Check sheet for the modelled part. Datum: model origin and axes. Units: mm. A direction names the side the tool comes from. Give positions to 0.01 mm unless a question says otherwise; leave off trailing zeros. Order: outer loops, then holes, each group sorted by start corner. A loop starts at its lowest first (then second) coordinate and runs counter-clockwise, first axis right, second up.
from build123d import *

# Parameters (mm, degrees)
IZIM1_R                     = 42
IZIM1_R_2                   = 40
Y_KSEKLIK_EKSTR_ZYON1_DEPTH = 15
IZIM2_R                     = 42
Y_KSEKLIK_EKSTR_ZYON2_DEPTH = 2
IZIM3_R                     = 1.75
KES_EKSTR_ZYON1_DEPTH       = 2
KES_EKSTR_ZYON2_DEPTH       = 2
Y_KSEKLIK_EKSTR_ZYON3_DEPTH = 7.5
Y_KSEKLIK_EKSTR_ZYON4_DEPTH = 35
Y_KSEKLIK_EKSTR_ZYON5_DEPTH = 4
Y_KSEKLIK_EKSTR_ZYON6_DEPTH = 4
IZIM9_W                     = 21
IZIM9_H                     = 3
Y_KSEKLIK_EKSTR_ZYON7_DEPTH = 45
IZIM10_R                    = 2.5
Y_KSEKLIK_EKSTR_ZYON8_DEPTH = 10
RADYUS1_R                   = 5


with BuildPart() as part:
    # Çizim1 → Yükseklik-Ekstrüzyon1 (new body)
    with BuildSketch(Plane(origin=(0, 0, 0), x_dir=(1, 0, 0), z_dir=(0, 1, 0))):
        with Locations(Location((0, 0, 0), (0, 0, 270))):
            Circle(IZIM1_R)
        with Locations(Location((0, 0, 0), (0, 0, 270))):
            Circle(IZIM1_R_2, mode=Mode.SUBTRACT)
    extrude(amount=Y_KSEKLIK_EKSTR_ZYON1_DEPTH)

    # Çizim2 → Yükseklik-Ekstrüzyon2 (add)
    with BuildSketch(Plane(origin=(0, 15, 0), x_dir=(1, 0, 0), z_dir=(0, 1, 0))):
        with Locations(Location((0, 0, 0), (0, 0, 270))):
            Circle(IZIM2_R)
    extrude(amount=Y_KSEKLIK_EKSTR_ZYON2_DEPTH)

    # Çizim3 → Kes-Ekstrüzyon1 (cut)
    with BuildSketch(Plane(origin=(0, 17, 0), x_dir=(1, 0, 0), z_dir=(0, 1, 0))):
        with Locations(Location((-13.5, 0, 0), (0, 0, 270))):
            Circle(IZIM3_R)
        with Locations(Location((13.5, 0, 0), (0, 0, 270))):
            Circle(IZIM3_R)
    extrude(amount=-KES_EKSTR_ZYON1_DEPTH, mode=Mode.SUBTRACT)

    # Çizim4 → Kes-Ekstrüzyon2 (cut)
    with BuildSketch(Plane(origin=(0, 17, 0), x_dir=(1, 0, 0), z_dir=(0, 1, 0))):
        with BuildLine():
            ThreePointArc((19.121323176, 19.121323176), (23.11330853, 20.564910887), (26.776285642, 18.419569137))
            ThreePointArc((26.776285642, 18.419569137), (30.026084807, -12.437211552), (5.909090909, -31.958295396))
            ThreePointArc((5.909090909, -31.958295396), (1.801989255, -30.88516514), (0, -27.041634566))
            ThreePointArc((0, -27.041634566), (1.156469426, -23.843623821), (4.090909091, -22.124973736))
            ThreePointArc((4.090909091, -22.124973736), (20.787289482, -8.610377228), (18.537428522, 12.752009403))
            ThreePointArc((18.537428522, 12.752009403), (17.677735465, 16.042240718), (19.121323176, 19.121323176))
        make_face()
    extrude(amount=-KES_EKSTR_ZYON2_DEPTH, mode=Mode.SUBTRACT)

    # Çizim5 → Yükseklik-Ekstrüzyon3 (add)
    with BuildSketch(Plane(origin=(0, 17, 0), x_dir=(1, 0, 0), z_dir=(0, 1, 0))):
        with BuildLine():
            Line((-10.5, -10), (-10.5, -2.645751311))
            ThreePointArc((-10.5, -2.645751311), (-9.5, 0), (-10.5, 2.645751311))
            Line((-10.5, 2.645751311), (-10.5, 18))
            Line((-10.5, 18), (10.5, 18))
            Line((10.5, 18), (10.5, 2.645751311))
            ThreePointArc((10.5, 2.645751311), (9.5, 0), (10.5, -2.645751311))
            Line((10.5, -2.645751311), (10.5, -10))
            Line((10.5, -10), (-10.5, -10))
        make_face()
    extrude(amount=Y_KSEKLIK_EKSTR_ZYON3_DEPTH)

    # Çizim6 → Yükseklik-Ekstrüzyon4 (add)
    with BuildSketch(Plane(origin=(0, 17, 0), x_dir=(1, 0, 0), z_dir=(0, 1, 0))):
        Polygon((-10.5, 18), (-10.5, 13), (-14.5, 13), (-14.5, 20), (-10.5, 20), align=None)
        Polygon((10.5, 20), (10.5, 18), (10.5, 13), (14.5, 13), (14.5, 20), align=None)
    extrude(amount=Y_KSEKLIK_EKSTR_ZYON4_DEPTH)

    # Çizim7 → Yükseklik-Ekstrüzyon5 (add)
    with BuildSketch(Plane(origin=(10.5, 0, 0), x_dir=(0, 0, -1), z_dir=(1, 0, 0))):
        Polygon((13, 52), (7.822875656, 17), (13, 17), align=None)
    extrude(amount=Y_KSEKLIK_EKSTR_ZYON5_DEPTH)

    # Çizim8 → Yükseklik-Ekstrüzyon6 (add)
    with BuildSketch(Plane.ZY.offset(10.5)):
        Polygon((-13, 52), (-7.822875656, 17), (-13, 17), align=None)
    extrude(amount=Y_KSEKLIK_EKSTR_ZYON6_DEPTH)

    # Çizim9 → Yükseklik-Ekstrüzyon7 (add)
    with BuildSketch(Plane(origin=(0, 17, 0), x_dir=(1, 0, 0), z_dir=(0, 1, 0))):
        with Locations((0, -16.5)):
            Rectangle(IZIM9_W, IZIM9_H)
    extrude(amount=Y_KSEKLIK_EKSTR_ZYON7_DEPTH)

    # Çizim10 → Yükseklik-Ekstrüzyon8 (add)
    with BuildSketch(Plane.XY.offset(18)):
        with Locations(Location((0, 54, 0), (0, 0, 180))):
            Circle(IZIM10_R)
    extrude(amount=Y_KSEKLIK_EKSTR_ZYON8_DEPTH)

    # Radyus1
    radyus1_edges = [part.edges().sort_by_distance(p)[0] for p in [
        (-10.5, 62, 16.5),
        (10.5, 62, 16.5),
    ]]
    fillet(radyus1_edges, radius=RADYUS1_R)


solid = part.part
1) Material ranges on L1, parallel to X at y = 16.25, z = 0; L2, parallel to X at y = 11.5, z = 0; L3, parallel to Y at x = 4.5, z = -11, recorded low to high.
Recorded:
L1: x = -42 to -15.25, -11.75 to 11.75, 15.25 to 22.5, 32.5 to 42
L2: x = -42 to -40, 40 to 42
L3: y = 15 to 24.5
2) Section check D-D, the plane x = -33. Record the cut outline in (y, z), then the cut area to 3 significant figures.
Recorded:
outline: (0, -25.98) - (17, -25.98) - (17, 25.98) - (0, 25.98) - (0, 22.61) - (15, 22.61) - (15, -22.61) - (0, -22.61) - close
area: 205 mm2
3) Section check A-A, the plane z = 0. Record the cut outline in (x, y), then the cut area to 4 significant figures.
Recorded:
outline: (-42, 0) - (-40, 0) - (-40, 15) - (-15.25, 15) - (-15.25, 17) - (-42, 17) - close; (-11.75, 15) - (11.75, 15) - (11.75, 17) - (9.5, 17) - (9.5, 24.5) - (-9.5, 24.5) - (-9.5, 17) - (-11.75, 17) - close; (15.25, 15) - (22.5, 15) - (22.5, 17) - (15.25, 17) - close; (32.5, 15) - (40, 15) - (40, 0) - (42, 0) - (42, 17) - (32.5, 17) - close
area: 336.5 mm2
4) Depth check by flat-ended pin: pin 1 Ø8 at (x, y) = (-1.5, 31.5) entering from -Z; pin 2 Ø6 at (y, z) = (19.5, 7) entering from -X; pin 3 Ø10.5 at (x, y) = (-3, 46.5) entering from +Z. Enter the tip coordinate at first touch or a pass-through.
Recorded:
pin 1: stops at z = 15
pin 2: stops at x = -41.66
pin 3: stops at z = 18
5) Set-up check for faces 1 (the face through (-10.5, 35, -16)), 2 (the face through (-13, 34, -20)), 3 (the face through (-10.5, 21, -6)), 4 (the face through (0, 54, 28)): record each of +Z, -Z, +X, -X, +Y, -Y from which the full face is reachable in a straight line by a thin tool's end or side.
Recorded:
face 1: -Z, +Y
face 2: -Z, +X, -X, +Y
face 3: +Z, -X, +Y
face 4: +Z, +X, -X, +Y
6) Draft check along Z on faces 5 (the face through (-12, 52, -17)), 6 (the face through (30.196, 16.014, 12.018)), 7 (the face through (-9.5, 20.7, 0)), 8 (the face through (12.472, 34.745, -10.448)). Enter one of: +Z half, -Z half, draft (parallel to the pull), parting line (faces both ways), or undercut.
Recorded:
face 5: draft
face 6: undercut
face 7: undercut
face 8: +Z half
7) Section check C-C, the plane y = 33. Record the cut outline in (x, z), then the cut area to 3 significant figures.
Recorded:
outline: (-14.5, -20) - (-10.5, -20) - (-10.5, -10.19) - (-14.5, -10.19) - close; (-10.5, 15) - (10.5, 15) - (10.5, 18) - (-10.5, 18) - close; (10.5, -20) - (14.5, -20) - (14.5, -10.19) - (10.5, -10.19) - close
area: 141 mm2
8) Section check B-B, the plane y = 54. Record the cut outline in (x, z).
Recorded:
outline: (-10.5, 15) - (10.5, 15) - (10.5, 18) - (2.5, 18) - (2.5, 28) - (-2.5, 28) - (-2.5, 18) - (-10.5, 18) - close
